```python
from build123d import *

# Parameters (mm, degrees)
SKETCH_3_R          = 2.55
SKETCH_3_R_2        = 1.55
EXTRUDE_1_DEPTH     = 5
SKETCH_4_R          = 1.55
EXTRUDE_2_DEPTH     = 9.25
FILLET_1_R          = 2
FILLET_START        = 6.9999999
FILLET_2_2_DEPTH    = 8.0000001
SKETCH_5_R          = 3
CUT_EXTRUDE_1_DEPTH = 2.5
SKETCH_6_R          = 7.55
CUT_EXTRUDE_2_DEPTH = 62.147874109


with BuildPart() as part:
    # 草图3 → 凸台-拉伸1 (new body)
    with BuildSketch(Plane.XY):
        with BuildLine():
            Line((13, 20), (34, 20))
            ThreePointArc((34, 20), (41.071067812, 17.071067812), (44, 10))
            Line((44, 10), (44, -10))
            ThreePointArc((44, -10), (41.071067812, -17.071067812), (34, -20))
            Line((34, -20), (13, -20))
            Line((13, -20), (-5, -9.797958971))
            ThreePointArc((-5, -9.797958971), (-11, 0), (-5, 9.797958971))
            Line((-5, 9.797958971), (13, 20))
        make_face()
        Circle(SKETCH_3_R, mode=Mode.SUBTRACT)
        with Locations((40.025, 8)):
            Circle(SKETCH_3_R_2, mode=Mode.SUBTRACT)
        with Locations((40.025, -8)):
            Circle(SKETCH_3_R_2, mode=Mode.SUBTRACT)
        with Locations((16.975, -8)):
            Circle(SKETCH_3_R_2, mode=Mode.SUBTRACT)
        with Locations((16.975, 8)):
            Circle(SKETCH_3_R_2, mode=Mode.SUBTRACT)
    extrude(amount=EXTRUDE_1_DEPTH)

    # 草图4 → 凸台-拉伸2 (add)
    with BuildSketch(Plane.XY.offset(5)):
        with BuildLine():
            Line((13, 20), (34, 20))
            ThreePointArc((34, 20), (41.071067812, 17.071067812), (44, 10))
            Line((44, 10), (44, -10))
            ThreePointArc((44, -10), (41.071067812, -17.071067812), (34, -20))
            Line((34, -20), (13, -20))
            Line((13, -20), (13, 20))
        make_face()
        with Locations((16.975, -8)):
            Circle(SKETCH_4_R, mode=Mode.SUBTRACT)
        with Locations((16.975, 8)):
            Circle(SKETCH_4_R, mode=Mode.SUBTRACT)
        with Locations((40.025, 8)):
            Circle(SKETCH_4_R, mode=Mode.SUBTRACT)
        with Locations((40.025, -8)):
            Circle(SKETCH_4_R, mode=Mode.SUBTRACT)
    extrude(amount=EXTRUDE_2_DEPTH)

    # 圆角1
    fillet_1_edges = [part.edges().sort_by_distance(p)[0] for p in [
        (13, 0, 5),
    ]]
    fillet(fillet_1_edges, radius=FILLET_1_R)

    # 圆角2: read off the stored shape, not the designer's step
    # 圆角2 outline → 圆角2 (revolve, cut)
    with BuildSketch(Plane(origin=(11, 0, 7), x_dir=(1, 0, 0), z_dir=(0, 0, 1))):
        with BuildLine():
            ThreePointArc((7, -20), (3.464466094, -18.535533906), (2, -15))
            Line((2, -15), (2, -20))
            Line((2, -20), (7, -20))
        make_face()
        with BuildLine():
            Line((2, 20), (2, 15))
            ThreePointArc((2, 15), (3.464466094, 18.535533906), (7, 20))
            Line((7, 20), (2, 20))
        make_face()
    revolve(axis=Axis((11, 0, 7), (0, 1, 0)), mode=Mode.SUBTRACT)

    # Fillet 2 2 outline → Fillet 2 2 (cut)
    with BuildSketch(Plane.XY.offset(FILLET_START)):
        with BuildLine():
            Line((13, -20), (18, -20))
            ThreePointArc((18, -20), (14.464466094, -18.535533906), (13, -15))
            Line((13, -15), (13, -20))
        make_face()
        with BuildLine():
            Line((13, 20), (13, 15))
            ThreePointArc((13, 15), (14.464466094, 18.535533906), (18, 20))
            Line((18, 20), (13, 20))
        make_face()
    extrude(amount=FILLET_2_2_DEPTH, mode=Mode.SUBTRACT)

    # 草图5 → 切除-拉伸1 (cut)
    with BuildSketch(Plane(origin=(0, 0, 0), x_dir=(-1, 0, 0), z_dir=(0, 0, -1))):
        with Locations((-40.025, 8)):
            Circle(SKETCH_5_R)
        with Locations((-16.975, 8)):
            Circle(SKETCH_5_R)
        with Locations((-16.975, -8)):
            Circle(SKETCH_5_R)
        with Locations((-40.025, -8)):
            Circle(SKETCH_5_R)
    extrude(amount=-CUT_EXTRUDE_1_DEPTH, mode=Mode.SUBTRACT)

    # 草图6 → 切除-拉伸2 (cut, through all)
    with BuildSketch(Plane.XZ.offset(20)):
        with Locations((28.5, 14.5)):
            Circle(SKETCH_6_R)
    extrude(amount=-CUT_EXTRUDE_2_DEPTH, mode=Mode.SUBTRACT)


solid = part.part
```
The model under review builds one solid part; all positions refer to its coordinate system, in mm. A direction names the side the tool comes from. Round coordinates to 2 decimals unless told otherwise and drop trailing zeros. Order: outer loops, then holes, each group sorted by start corner. A loop starts at its lowest first (then second) coordinate and runs counter-clockwise, first axis right, second up.
(1) Take a section at B-B, the plane z = 8.5. State the section outline as (x, y) points (3 decimals).
Working result:
outline: (13, -15) arc R5 ccw to (18, -20) - (23.917, -20) - (23.917, 20) - (18, 20) arc R5 ccw to (13, 15) - close; (33.083, -20) - (34, -20) arc R10 ccw to (44, -10) - (44, 10) arc R10 ccw to (34, 20) - (33.083, 20) - close; hole circle Ø3.1 at (16.975, -8); hole circle Ø3.1 at (16.975, 8); hole circle Ø3.1 at (40.025, -8); hole circle Ø3.1 at (40.025, 8)
(2) Mouldability with a two-part tool opening along Y and no side actions: class faces 4 (the face through (28.34, -0.28, 6.95)), 5 (the face through (19.972, 8.132, 1.232)), 6 (the face through (4.126, -14.97, 2.465)) as released by +Y, released by -Y, zero draft, split by the parting line, or undercut.
Working result:
face 4: zero draft
face 5: undercut
face 6: released by -Y
(3) Wall thickness on L1, parallel to X at y = -8, z = 8.25 (3 decimals); L2, parallel to X at y = 9.5, z = 2; L3, parallel to X at y = -8, z = 7.5 (3 decimals): over which ranges is each line inside the solid? List them lowest first.
Working result:
L1: x = 13 to 15.425, 18.525 to 24.264, 32.736 to 38.475, 41.575 to 44
L2: x = -5.55 to 14.38, 19.57 to 37.43, 42.62 to 44
L3: x = 13 to 15.425, 18.525 to 25.671, 31.329 to 38.475, 41.575 to 44
(4) Tool access review of faces 1 (the face through (3, 0, 5)), 2 (the face through (14, 18, 11)), 3 (the face through (19.972, -7.868, 1.232)): name each direction out of +Z, -Z, +X, -X, +Y, -Y from which nothing blocks a thin tool from reaching the whole face with its end or side.
Working result:
face 1: +Z, -X, +Y, -Y
face 2: +Z, -X, +Y
face 3: -Z
(5) For P1, Ø6, axis at y = 4, z = 12.5, coming from the -X side; P2, Ø4, axis at x = 32.5, y = -13, coming from the +Z side; P3, Ø2, axis at y = -12, z = 5, coming from the +X side; P4, Ø1.9, axis at x = 16.975, y = 8, coming from the +Z side, all flat-tipped, find the tip position at first contact; note any pin that passes through.
Working result:
P1: stops at x = 13
P2: stops at z = 9.92
P3: stops at x = 43.95
P4: passes through
(6) Take a section at D-D, the plane y = 8. State the section outline as (x, z) points (3 decimals), plus the area to 3 significant figures.
Working result:
outline: (-7.55, 0) - (13.975, 0) - (13.975, 2.5) - (15.425, 2.5) - (15.425, 14.25) - (13, 14.25) - (13, 7) arc R2 cw to (11, 5) - (-7.55, 5) - close; (18.525, 2.5) - (19.975, 2.5) - (19.975, 0) - (37.025, 0) - (37.025, 2.5) - (38.475, 2.5) - (38.475, 14.25) - (36.046, 14.25) arc R7.55 cw to (20.954, 14.25) - (18.525, 14.25) - close; (41.575, 2.5) - (43.025, 2.5) - (43.025, 0) - (44, 0) - (44, 14.25) - (41.575, 14.25) - close
area: 357 mm2
(7) Take a section at C-C, the plane x = 0. State the section outline as (y, z) points.
Working result:
outline: (-12.63, 0) - (-2.55, 0) - (-2.55, 5) - (-12.63, 5) - close; (2.55, 0) - (12.63, 0) - (12.63, 5) - (2.55, 5) - close
